The drawing under review shows one solid part. Ordinate dimensions are in mm from its lowest x, y, z. Coordinates: 2 decimals unless noted, no trailing zeros. Loops run counter-clockwise (first coordinate to the right, second up) from the corner with the lowest first, then second, coordinate; pieces in that order, holes last. Notation, with made-up numbers: M 59,47 L 116,47 A21 ccw 116,70 Z; hole C -1.5,65 d5. An arc over 180 degrees is marked long. Use one line per item in the form item = value.
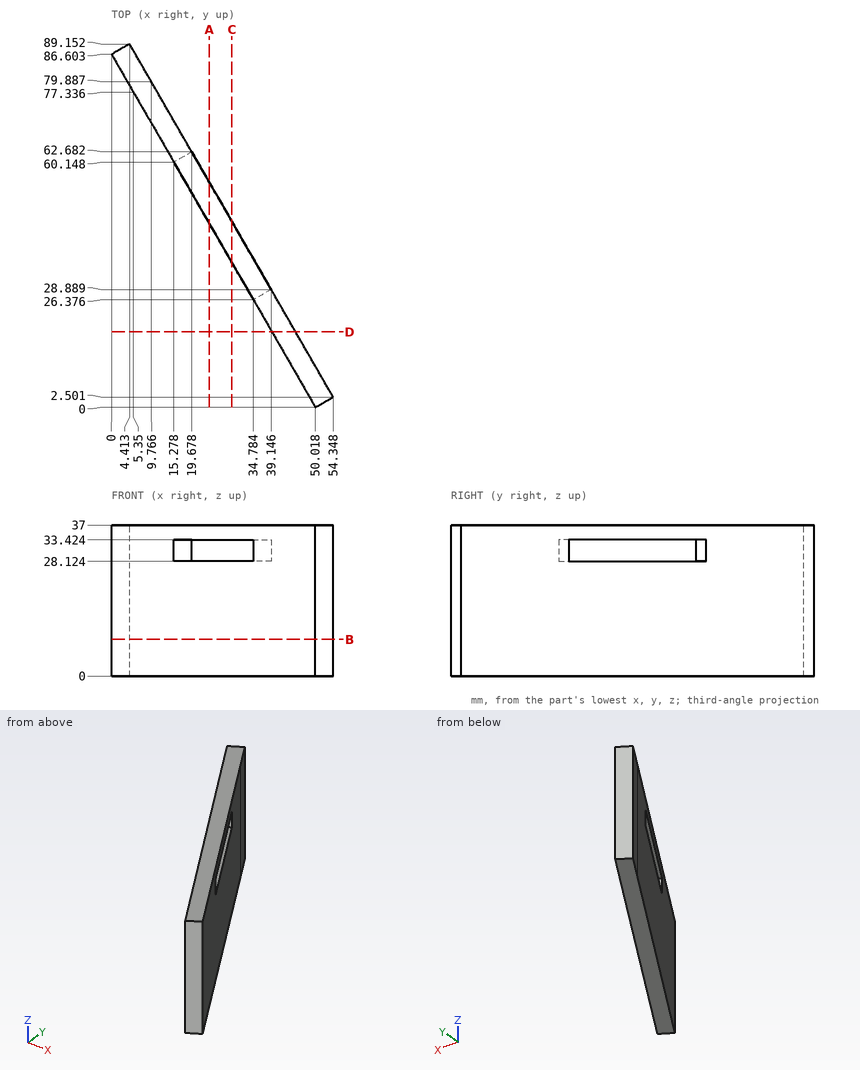
1. Consider section A-A on x = 24. Write out the cut boundary in (y, z) (1 decimal), plus the area to 3 significant figures.
Computed values:
outline = M 45,0 L 55.2,0 L 55.2,28.1 L 45,28.1 Z; M 45,33.4 L 55.2,33.4 L 55.2,37 L 45,37 Z
area = 321 mm2
2. Consider section B-B on z = 9. Write out the cut boundary in (x, y).
Computed values:
outline = M 0,86.6 L 5.35,77.34 L 50.02,0 L 54.35,2.5 L 9.77,79.89 L 4.41,89.15 Z
3. Wall thickness on line 1 along Z through (x, y) = (27, 46.5) (1 decimal); line 2 along X through (y, z) = (33, 2); line 3 along X through (y, z) = (29.5, 22) (1 decimal): over which ranges is each line inside the solid? List them lowest first. Write a range as from..to.
Computed values:
line_1 = 0..28.1, 33.4..37
line_2 = 30.96..36.78
line_3 = 33..38.8
4. Consider section D-D on y = 18.5. Write out the cut boundary in (x, z).
Computed values:
outline = M 39.33,0 L 45.13,0 L 45.13,37 L 39.33,37 Z
5. Consider section C-C on x = 29.5. Write out the cut boundary in (y, z) (1 decimal).
Computed values:
outline = M 35.5,0 L 45.6,0 L 45.6,28.1 L 35.5,28.1 Z; M 35.5,33.4 L 45.6,33.4 L 45.6,37 L 35.5,37 Z
6. For pin 1 Ø5 at (y, z) = (66.5, 25.5) entering from -X (1 decimal); pin 2 Ø8 at (x, z) = (34, 30.5) entering from +Y (1 decimal); pin 3 Ø1.5 at (y, z) = (79, 32) entering from -X, all flat-tipped, find the tip position at first contact; note any pin that passes through.
Computed values:
pin_1 = 10.2
pin_2 = 43.4
pin_3 = 3.96
